CAD build for the part. Positions are in the model's coordinates, mm. A direction names the side the tool comes from. Round coordinates to 2 decimals unless told otherwise and drop trailing zeros. Order: outer loops, then holes, each group sorted by start corner. A loop starts at its lowest first (then second) coordinate and runs counter-clockwise, first axis right, second up. Notation, with made-up numbers: (41.5, 79) - (90.5, 79) arc R25 ccw to (90.5, 99) - close; hole circle Ø11 at (-7.5, 60.25). An arc over 180 degrees is marked (long way). Use one line per item in the form item = value. Start each with the question number.
from build123d import *


with BuildPart() as f1:
    # F0 (on Front) → F1 (revolve)
    with BuildSketch(Plane.XZ):
        with BuildLine():
            Line((0, -67.055455), (0, 45.944545))
            Line((0, 45.944545), (-2.5, 45.944545))
            Line((-2.5, 45.944545), (-2.5, 40.944545))
            Line((-2.5, 40.944545), (-1.342105, 40.944545))
            Line((-1.342105, 40.944545), (-1.342105, 35.944545))
            Line((-1.342105, 35.944545), (-2.5, 35.944545))
            Line((-2.5, 35.944545), (-2.5, 20.944545))
            Line((-2.5, 20.944545), (-4.25, 20.944545))
            Line((-4.25, 20.944545), (-4.25, -7.055455))
            ThreePointArc((-4.25, -7.055455), (-10.591536, -9.772009), (-13, -16.23684))
            Line((-13, -16.23684), (-13, -38.544123))
            Line((-13, -38.544123), (-11.674659, -39.383397))
            Line((-11.674659, -39.383397), (-11.674659, -52.055455))
            Line((-11.674659, -52.055455), (-13, -52.055455))
            Line((-13, -52.055455), (-13, -54.909937))
            Line((-13, -54.909937), (-9.052842, -67.055455))
            Line((-9.052842, -67.055455), (0, -67.055455))
        make_face()
    revolve(axis=Axis((0, 0, -10.555455), (0, 0, 1)))


solid = f1.part
(1) Slice it at B-B (z = -24.5). Give the cut face in (x, y).
(2) Which spindle directions (+Z, -Z, +X, -X, +Y, -Y) get a long thin tool onto all of the face, cutting with end or side? Do faces 4 (the cylindrical face through (0.54, 2.44, 43.41)), 5 (the cylindrical face through (10.316, 7.91, -53.503)), 6 (the cylindrical face through (-11.136, -3.507, -45.808)). Say none if no direction does.
(3) Wall check: line 1 (X direction, y = 0, z = 35.5); line 2 (Y direction, x = 2.5, z = 7); line 3 (X direction, y = -6.75, z = -50.5). Give the ranges that are in metal, low to high. Write a range as [from, to].
(4) Flat gauge pins, fed straight in: P1, Ø1.5, axis at y = -3, z = 25, coming from the -X side; P2, Ø10, axis at x = -9, y = 3.5, coming from the -Z side; P3, Ø1.5, axis at x = 7, y = -3.5, coming from the +Z side; P4, Ø2, axis at y = 1.5, z = 3, coming from the +X side. Where does each tip first touch, or does it go through?
(5) Mould opens along Z. For faces 1 (the flat face through (0, 0, -67.055)), 2 (the cylindrical face through (10.316, 7.91, -27.547)), 3 (the cylindrical face through (1.065, 0.817, 38.41)) say: pulls with the +Z half, pulls with the -Z half, needs draft (parallel to the pull), parting line crosses it, or undercut.
(6) Slice it at A-A (z = -51). Give the cut face in (x, y).
Results list:
q1.outline = circle Ø26 at (0, 0)
q2.face_4 = +Z
q2.face_5 = +Z, -Z
q2.face_6 = none
q3.line_1 = [-2.5, 2.5]
q3.line_2 = [-3.44, 3.44]
q3.line_3 = [-9.53, 9.53]
q4.P1 = -1.09
q4.P2 = -67.06
q4.P3 = -7.52
q4.P4 = 4.22
q5.face_1 = pulls with the -Z half
q5.face_2 = needs draft
q5.face_3 = undercut
q6.outline = circle Ø23.35 at (0, 0)
